from build123d import *

# Parameters (mm, degrees)
RESSALTO_EXTRUS_O1_DEPTH = 4
FURO_COM_FOLGA_DE_M31_D  = 3.2
FILETE1_R                = 3
M3_CLEARANCE_HOLE1_D     = 3.2
FURO_COM_FOLGA_DE_M32_D  = 2.87
M3_CLEARANCE_HOLE2_D     = 3.2
SKETCH3_W                = 27.430623534
SKETCH3_H                = 190
CUT_EXTRUDE1_DEPTH       = 10
BOSS_EXTRUDE1_DEPTH      = 4
CUT_EXTRUDE3_DEPTH       = 10
FILLET2_R                = 3
FILLET3_R                = 3
SKETCH9_W                = 23.417498706
SKETCH9_H                = 10.613187714
SKETCH9_W_2              = 56.748489153
BOSS_EXTRUDE2_DEPTH      = 4
FILLET4_R                = 3
BOSS_EXTRUDE3_DEPTH      = 4
M3_CLEARANCE_HOLE4_D     = 3.2
FILLET5_R                = 3
M5_CLEARANCE_HOLE1_D     = 5.3
CUT_EXTRUDE4_DEPTH       = 215.251953603
CUT_EXTRUDE5_DEPTH       = 215.251953603
SKETCH15_R               = 5.5
CUT_EXTRUDE6_DEPTH       = 215.251953603
M5_CLEARANCE_HOLE2_D     = 5.3
FILLET6_R                = 3


# Some blends are built 0.0001 mm under size
with BuildPart() as part:
    # Esboço1 → Ressalto-extrusão1 (new body)
    with BuildSketch(Plane.XY):
        with BuildLine():
            Line((168.243612151, -138.115636704), (-79.756387849, -138.115636704))
            ThreePointArc((-79.756387849, -138.115636704), (-80.46349463, -137.822743485), (-80.756387849, -137.115636704))
            Line((-80.756387849, -137.115636704), (-80.756387849, 48.884363296))
            ThreePointArc((-80.756387849, 48.884363296), (-79.877708192, 51.005683639), (-77.756387849, 51.884363296))
            Line((-77.756387849, 51.884363296), (166.243612151, 51.884363296))
            ThreePointArc((166.243612151, 51.884363296), (168.364932495, 51.005683639), (169.243612151, 48.884363296))
            Line((169.243612151, 48.884363296), (169.243612151, -137.115636704))
            ThreePointArc((169.243612151, -137.115636704), (168.950718933, -137.822743485), (168.243612151, -138.115636704))
        make_face()
        with BuildLine():
            Line((-36.756387849, -93.115636704), (-55.756387849, -93.115636704))
            Line((-55.756387849, -93.115636704), (-55.756387849, -79.115636704))
            Line((-55.756387849, -79.115636704), (-55.756387849, 27.884363296))
            ThreePointArc((-55.756387849, 27.884363296), (-54.877708192, 30.005683639), (-52.756387849, 30.884363296))
            Line((-52.756387849, 30.884363296), (141.243612151, 30.884363296))
            ThreePointArc((141.243612151, 30.884363296), (143.364932495, 30.005683639), (144.243612151, 27.884363296))
            Line((144.243612151, 27.884363296), (144.243612151, -79.115636704))
            Line((144.243612151, -79.115636704), (144.243612151, -93.115636704))
            Line((144.243612151, -93.115636704), (125.243612151, -93.115636704))
            Line((125.243612151, -93.115636704), (125.243612151, -118.115636704))
            ThreePointArc((125.243612151, -118.115636704), (124.950718933, -118.822743485), (124.243612151, -119.115636704))
            Line((124.243612151, -119.115636704), (-35.756387849, -119.115636704))
            ThreePointArc((-35.756387849, -119.115636704), (-36.46349463, -118.822743485), (-36.756387849, -118.115636704))
            Line((-36.756387849, -118.115636704), (-36.756387849, -93.115636704))
        make_face(mode=Mode.SUBTRACT)
    extrude(amount=RESSALTO_EXTRUS_O1_DEPTH)

    # Furo com folga de M31 (through all)
    with Locations(Plane(origin=(0, 0, 0), x_dir=(-1, 0, 0), z_dir=(0, 0, -1))):
        with Locations((-148.743612151, -78.347886704), (-148.743612151, -18.347886704), (-148.743612151, 41.652113296), (60.256387849, 41.652113296), (60.256387849, -18.347886704), (60.256387849, -78.347886704)):
            Hole(FURO_COM_FOLGA_DE_M31_D / 2)

    # Filete1
    filete1_edges = [part.edges().sort_by_distance(p)[0] for p in [
        (-55.756387849, -93.115636704, 2),
        (-36.756387849, -93.115636704, 2),
        (125.243612151, -93.115636704, 2),
        (144.243612151, -93.115636704, 2),
    ]]
    fillet(filete1_edges, radius=FILETE1_R)

    # M3 Clearance Hole1 (through all)
    with Locations(Plane(origin=(0, 0, 0), x_dir=(-1, 0, 0), z_dir=(0, 0, -1))):
        with Locations((-164.230041881, -97.102981335), (43.669958119, -97.102981335), (75.742817578, -97.102981335)):
            Hole(M3_CLEARANCE_HOLE1_D / 2)

    # Furo com folga de M32 (through all)
    with Locations(Plane.XY.offset(4)):
        with Locations((44.243612151, 46.98714614)):
            Hole(FURO_COM_FOLGA_DE_M32_D / 2)

    # M3 Clearance Hole2 (through all)
    with Locations(Plane.XY.offset(4)):
        with Locations((161.560317261, 35.480164232), (161.560317261, 4.480164232)):
            Hole(M3_CLEARANCE_HOLE2_D / 2)

    # Sketch3 → Cut-Extrude1 (cut)
    with BuildSketch(Plane.XY.offset(4)):
        with Locations((169.958923918, -43.115636704)):
            Rectangle(SKETCH3_W, SKETCH3_H)
    extrude(amount=-CUT_EXTRUDE1_DEPTH, mode=Mode.SUBTRACT)

    # Sketch5 → Boss-Extrude1 (add)
    with BuildSketch(Plane(origin=(0, 0, 0), x_dir=(-1, 0, 0), z_dir=(0, 0, -1))):
        with BuildLine():
            Line((-145.240285588, -97.500155699), (-140.243612151, -97.500155699))
            Line((-140.243612151, -97.500155699), (-140.243612151, 27.941506315))
            ThreePointArc((-140.243612151, 27.941506315), (-139.345176367, 30.025791601), (-137.244155982, 30.884363296))
            Line((-137.244155982, 30.884363296), (-145.240285588, 30.884363296))
            Line((-145.240285588, 30.884363296), (-145.240285588, -97.500155699))
        make_face()
    extrude(amount=-BOSS_EXTRUDE1_DEPTH)

    # Sketch6 → Cut-Extrude3 (cut)
    with BuildSketch(Plane(origin=(0, 0, 0), x_dir=(-1, 0, 0), z_dir=(0, 0, -1))):
        with BuildLine():
            Line((-108.923612151, -113.115636704), (-128.243612151, -113.115636704))
            Line((-128.243612151, -113.115636704), (-128.243612151, -98.115636704))
            ThreePointArc((-128.243612151, -98.115636704), (-129.708078246, -94.580102798), (-133.243612151, -93.115636704))
            Line((-133.243612151, -93.115636704), (44.756387849, -93.115636704))
            ThreePointArc((44.756387849, -93.115636704), (41.220853943, -94.580102798), (39.756387849, -98.115636704))
            Line((39.756387849, -98.115636704), (39.756387849, -113.115636704))
            Line((39.756387849, -113.115636704), (20.436387849, -113.115636704))
            Line((20.436387849, -113.115636704), (20.436387849, -119.115636704))
            Line((20.436387849, -119.115636704), (-108.923612151, -119.115636704))
            Line((-108.923612151, -119.115636704), (-108.923612151, -113.115636704))
        make_face()
    extrude(amount=-CUT_EXTRUDE3_DEPTH, mode=Mode.SUBTRACT)

    # Fillet2
    fillet2_edges = [part.edges().sort_by_distance(p)[0] for p in [
        (-39.756387849, -113.115636704, 2),
        (128.243612151, -113.115636704, 2),
        (140.243612151, -93.115636704, 2),
    ]]
    fillet(fillet2_edges, radius=FILLET2_R - 0.0001)  # a hair under: the kernel refuses the full size

    # Fillet3
    fillet3_edges = [part.edges().sort_by_distance(p)[0] for p in [
        (156.243612151, 51.884363296, 2),
    ]]
    fillet(fillet3_edges, radius=FILLET3_R)

    # Sketch9 → Boss-Extrude2 (add)
    with BuildSketch(Plane(origin=(0, 0, 0), x_dir=(-1, 0, 0), z_dir=(0, 0, -1))):
        with Locations((-117.632361503, -114.422230557)):
            Rectangle(SKETCH9_W, SKETCH9_H)
        with Locations((12.794195261, -114.422230557)):
            Rectangle(SKETCH9_W_2, SKETCH9_H)
    extrude(amount=-BOSS_EXTRUDE2_DEPTH)

    # Fillet4
    fillet4_edges = [part.edges().sort_by_distance(p)[0] for p in [
        (105.92361215, -119.115636704, 2),
        (105.92361215, -109.1156367, 2),
        (15.580049316, -119.115636704, 2),
        (15.580049316, -109.1156367, 2),
    ]]
    fillet(fillet4_edges, radius=FILLET4_R)

    # Sketch10 → Boss-Extrude3 (add)
    with BuildSketch(Plane(origin=(0, 0, 0), x_dir=(-1, 0, 0), z_dir=(0, 0, -1))):
        with BuildLine():
            Line((-156.243612151, -135.615636704), (-160.743612151, -135.615636704))
            ThreePointArc((-160.743612151, -135.615636704), (-163.743612151, -132.615636704), (-160.743612151, -129.615636704))
            Line((-160.743612151, -129.615636704), (-156.243612151, -129.615636704))
            Line((-156.243612151, -129.615636704), (-156.243612151, -135.615636704))
        make_face()
        with BuildLine():
            Line((-156.243612151, -98.615636704), (-160.743612151, -98.615636704))
            ThreePointArc((-160.743612151, -98.615636704), (-163.743612151, -101.615636704), (-160.743612151, -104.615636704))
            Line((-160.743612151, -104.615636704), (-156.243612151, -104.615636704))
            Line((-156.243612151, -104.615636704), (-156.243612151, -98.615636704))
        make_face()
    extrude(amount=-BOSS_EXTRUDE3_DEPTH)

    # M3 Clearance Hole4 (through all)
    with Locations(Plane(origin=(0, 0, 0), x_dir=(-1, 0, 0), z_dir=(0, 0, -1))):
        with Locations((-160.743612151, -101.615636704), (-160.743612151, -132.615636704), (-129.743612151, -132.615636704)):
            Hole(M3_CLEARANCE_HOLE4_D / 2)

    # Fillet5
    # the kernel refuses this fillet: 3 mm, written as the material it adds along each edge
    with BuildSketch(Plane(origin=(156.243612151, -129.615636704, 0), x_dir=(0, 1, 0), z_dir=(0, 0, 1)), Plane(origin=(156.243612151, -98.615636704, 0), x_dir=(0, 1, 0), z_dir=(0, 0, 1)), Plane(origin=(156.243612151, -104.615636704, 0), x_dir=(1, 0, 0), z_dir=(0, 0, 1))) as fillet5_piece_1:
        with BuildLine():
            CenterArc((FILLET5_R, -FILLET5_R), FILLET5_R, 90, 90)
            Line((0, -FILLET5_R), (-FILLET5_R * 0.02, -FILLET5_R))
            Line((-FILLET5_R * 0.02, -FILLET5_R), (-FILLET5_R * 0.02, FILLET5_R * 0.02))
            Line((-FILLET5_R * 0.02, FILLET5_R * 0.02), (FILLET5_R, FILLET5_R * 0.02))
            Line((FILLET5_R, FILLET5_R * 0.02), (FILLET5_R, 0))
        make_face()
    extrude(amount=4)
    with BuildSketch(Plane(origin=(156.243612151, -135.615636704, 0), x_dir=(0, -1, 0), z_dir=(0, 0, 1))) as fillet5_piece_2:
        with BuildLine():
            CenterArc((3, 2.958039892), FILLET5_R, 180, 80.405931773)
            Line((0, 2.958039892), (-0.06, 2.958039892))
            Line((-0.06, 2.958039892), (-0.06, 0))
            Line((-0.06, 0), (0, -0.06))
            ThreePointArc((0, -0.06), (1.25, -0.06), (2.49, -0.059160798))
            Line((2.49, -0.059160798), (2.5, 0))
        make_face()
    extrude(amount=4)

    # M5 Clearance Hole1 (through all)
    with Locations(Plane(origin=(0, 0, 0), x_dir=(-1, 0, 0), z_dir=(0, 0, -1))):
        with Locations((-115.03361215, -121.8656367), (26.54638785, -121.8656367)):
            Hole(M5_CLEARANCE_HOLE1_D / 2)

    # Sketch13 → Cut-Extrude4 (cut, through all)
    with BuildSketch(Plane.XY.offset(4)):
        with BuildLine():
            Line((-4.670217718, -138.115636704), (-37.787747523, -138.115636704))
            Line((-37.787747523, -138.115636704), (-37.787747523, -136.092387065))
            ThreePointArc((-37.787747523, -136.092387065), (-37.201961086, -134.678173503), (-35.787747523, -134.092387065))
            Line((-35.787747523, -134.092387065), (-6.670217718, -134.092387065))
            ThreePointArc((-6.670217718, -134.092387065), (-5.256004156, -134.678173503), (-4.670217718, -136.092387065))
            Line((-4.670217718, -136.092387065), (-4.670217718, -138.115636704))
        make_face()
        with BuildLine():
            Line((126.398542328, -138.115636704), (93.281012523, -138.115636704))
            Line((93.281012523, -138.115636704), (93.281012523, -136.092387065))
            ThreePointArc((93.281012523, -136.092387065), (93.866798961, -134.678173503), (95.281012523, -134.092387065))
            Line((95.281012523, -134.092387065), (124.398542328, -134.092387065))
            ThreePointArc((124.398542328, -134.092387065), (125.812755891, -134.678173503), (126.398542328, -136.092387065))
            Line((126.398542328, -136.092387065), (126.398542328, -138.115636704))
        make_face()
    extrude(amount=-CUT_EXTRUDE4_DEPTH, mode=Mode.SUBTRACT)

    # Sketch14 → Cut-Extrude5 (cut, through all)
    with BuildSketch(Plane.XY.offset(4)):
        with BuildLine():
            Line((47.021220635, -124.115636704), (51.521220635, -124.115636704))
            ThreePointArc((51.521220635, -124.115636704), (55.521220635, -128.115636704), (51.521220635, -132.115636704))
            Line((51.521220635, -132.115636704), (47.021220635, -132.115636704))
            ThreePointArc((47.021220635, -132.115636704), (43.021220635, -128.115636704), (47.021220635, -124.115636704))
        make_face()
    extrude(amount=-CUT_EXTRUDE5_DEPTH, mode=Mode.SUBTRACT)

    # Sketch15 → Cut-Extrude6 (cut, through all)
    with BuildSketch(Plane(origin=(0, 0, 0), x_dir=(-1, 0, 0), z_dir=(0, 0, -1))):
        with Locations((-144.771180456, -129.756932302)):
            Circle(SKETCH15_R)
        with Locations((-145.243612151, -117.115636704)):
            Circle(SKETCH15_R)
    extrude(amount=-CUT_EXTRUDE6_DEPTH, mode=Mode.SUBTRACT)

    # M5 Clearance Hole2 (through all)
    with Locations(Plane.XY.offset(4)):
        with Locations((-6.93638785, -119.870636704), (8.06361215, -119.870636704)):
            Hole(M5_CLEARANCE_HOLE2_D / 2)

    # Fillet6
    fillet6_edges = [part.edges().sort_by_distance(p)[0] for p in [
        (128.243612151, -109.1156367, 2),
        (-39.756387849, -109.1156367, 2),
    ]]
    fillet(fillet6_edges, radius=FILLET6_R)


solid = part.part
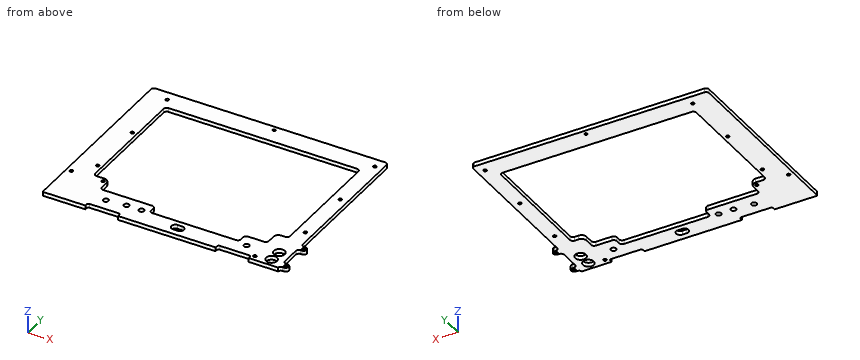
Here's how the part is built. I have some questions about the finished solid (model axes, mm). Coordinates: 2 decimals unless noted, no trailing zeros. Write each loop counter-clockwise with the first axis right and the second up, starting at its lowest first coordinate (ties: lowest second). Pieces come first, ordered by that corner, then holes. Notation, with made-up numbers: (-26.75, 44.5) - (-3.75, 44.5) arc R30 ccw to (-3.75, 78.5) - close; hole circle Ø2 at (20, -21.75). An arc over 180 degrees is marked (long way). Use one line per item in the form item = value.
1) I'm going to push flat-ended pins straight in: P1, Ø12.5, axis at x = 145.24, y = -117.12, coming from the -Z side; P2, Ø2, axis at x = 111.5, z = 2.5, coming from the -Y side; P3, Ø1.2, axis at x = 159.5, z = 1.5, coming from the -Y side. Where does each tip first touch, or does it pass through?
Solved:
P1 = 0
P2 = -134.09
P3 = -135.63
2) Suppose I cut it at B-B, the plane x = 77.5. Write out the boundary of the cut face in (y, z).
Solved:
outline = (-138.12, 0) - (-119.12, 0) - (-119.12, 4) - (-138.12, 4) - close; (30.88, 0) - (51.88, 0) - (51.88, 4) - (30.88, 4) - close
3) Suppose I cut it at A-A, the plane y = 0. Write out the boundary of the cut face in (x, z), plus the area to 3 significant figures.
Solved:
outline = (-80.76, 0) - (-55.76, 0) - (-55.76, 4) - (-80.76, 4) - close; (140.24, 0) - (156.24, 0) - (156.24, 4) - (140.24, 4) - close
area = 164 mm2
4) I need wall thicknesses on line 1 (X direction, y = 11, z = 2.55); line 2 (Y direction, x = -51.5, z = 3.1); line 3 (Y direction, x = 42.5, z = 3.4). Which ranges of each line are inside material? Lowest first, please.
Solved:
line_1 = -80.76 to -55.76, 140.24 to 156.24
line_2 = -138.12 to -93.12, 30.88 to 51.88
line_3 = -138.12 to -119.12, 30.88 to 51.88
5) Suppose I cut it at D-D, the plane z = 1.95. Give the number of separate pieces and of enclosed holes in the cut face, plus the area to 3 significant figures.
Solved:
separate_pieces = 1
enclosed_holes = 20
area = 16,500 mm2
6) Suppose I cut it at C-C, the plane x = 115. Write out the boundary of the cut face in (y, z), plus the area to 3 significant figures.
Solved:
outline = (-134.09, 0) - (-124.52, 0) - (-124.52, 4) - (-134.09, 4) - close; (-119.22, 0) - (-109.12, 0) - (-109.12, 4) - (-119.22, 4) - close; (30.88, 0) - (51.88, 0) - (51.88, 4) - (30.88, 4) - close
area = 163 mm2
